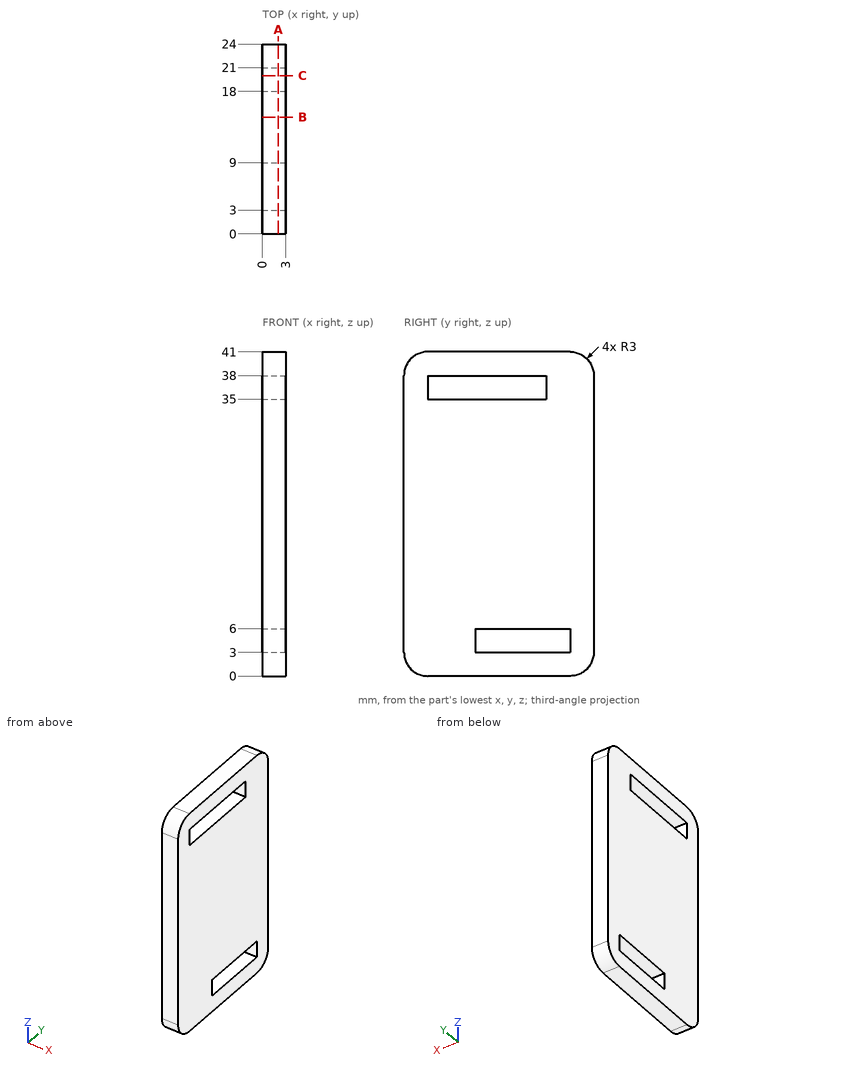
Input: dimensioned drawing with shaded views. Units: mm. Origin: part minimum x, y, z. Round coordinates to 2 decimals unless told otherwise and drop trailing zeros. Loops run counter-clockwise (first coordinate to the right, second up) from the corner with the lowest first, then second, coordinate; pieces in that order, holes last. Notation, with made-up numbers: (-28, 59.5) -> (5, 59.5) arc R30 ccw to (5, 96.5) -> close; hole circle Ø6 at (10.25, 32.25). An arc over 180 degrees is marked (long way). Answer as a JSON object with one key per item and string values. Group by question number.
1) Section query B-B on y = 14.75. Output: boundary loops of the cut face in (x, z).
2) Ray query, L1, parallel to Z at x = 0.35, y = 14.25; L2, parallel to Y at x = 1.85, z = 37.5; L3, parallel to Z at x = 1.45, y = 18.75. Return the intervals inside material, ascending.
3) Section query C-C on y = 20. Output: boundary loops of the cut face in (x, z).
4) Section query A-A on x = 2.05. Output: boundary loops of the cut face in (y, z), plus the area to 3 significant figures.
5) Pin query (flat end, axial travel): pin 1 (0.9 mm diameter, centred on x = 1, z = 36, fed in from -Y). Return the tip coordinate at first contact, or that it passes through.
Reply:
{
 "1": {"outline": "(0, 0) -> (3, 0) -> (3, 3) -> (0, 3) -> close; (0, 6) -> (3, 6) -> (3, 35) -> (0, 35) -> close; (0, 38) -> (3, 38) -> (3, 41) -> (0, 41) -> close"},
 "2": {"L1": "z = 0 to 3, 6 to 35, 38 to 41", "L2": "y = 0 to 3, 18 to 24", "L3": "z = 0 to 3, 6 to 41"},
 "3": {"outline": "(0, 0) -> (3, 0) -> (3, 3) -> (0, 3) -> close; (0, 6) -> (3, 6) -> (3, 41) -> (0, 41) -> close"},
 "4": {"outline": "(0, 3) arc R3 ccw to (3, 0) -> (21, 0) arc R3 ccw to (24, 3) -> (24, 38) arc R3 ccw to (21, 41) -> (3, 41) arc R3 ccw to (0, 38) -> close; hole (3, 35) -> (18, 35) -> (18, 38) -> (3, 38) -> close; hole (9, 3) -> (21, 3) -> (21, 6) -> (9, 6) -> close", "area": "895 mm2"},
 "5": {"pin 1": "stops at y = 0"}
}
